from build123d import *

# Parameters (mm, degrees)
SKETCH1_W               = 355.6
SKETCH1_H               = 50.8
BOSS_EXTRUDE1_DEPTH     = 3.175
SKETCH2_W               = 38.1
SKETCH2_H               = 3.175
BOSS_EXTRUDE2_DEPTH     = 3.175
MIRROR2_COPY_1_SKETCH_W = 38.1
MIRROR2_COPY_1_SKETCH_H = 3.175
MIRROR2_COPY_1_DEPTH    = 3.175
SKETCH3_W               = 3.302
SKETCH3_H               = 26.67
CUT_EXTRUDE1_DEPTH      = 3.175
SKETCH4_R               = 1.4732
SKETCH4_R_2             = 12
SKETCH4_W               = 12.192
SKETCH4_H               = 12.192
CUT_EXTRUDE2_DEPTH      = 1
CUT_EXTRUDE2_DEPTH_BACK = 4.175


with BuildPart() as part:
    # Sketch1 → Boss-Extrude1 (new body)
    with BuildSketch(Plane.XY):
        with Locations((177.8, 25.4)):
            Rectangle(SKETCH1_W, SKETCH1_H)
    extrude(amount=BOSS_EXTRUDE1_DEPTH)

    # Sketch2 → Boss-Extrude2 (add)
    with BuildSketch(Plane(origin=(0, 50.8, 0), x_dir=(1, 0, 0), z_dir=(0, 1, 0))):
        with Locations((50.8, -1.5875)):
            Rectangle(SKETCH2_W, SKETCH2_H)
        with Locations((127, -1.5875)):
            Rectangle(SKETCH2_W, SKETCH2_H)
    boss_extrude2 = extrude(amount=BOSS_EXTRUDE2_DEPTH)

    # Mirror1: Boss-Extrude2 across plane
    add(boss_extrude2.mirror(Plane.ZY.offset(-177.8)))

    # Mirror2: Boss-Extrude2 across plane
    add(boss_extrude2.mirror(Plane.ZX.offset(25.4)))

    # Mirror2 copy 1 sketch → Mirror2 copy 1 (add)
    with BuildSketch(Plane(origin=(355.6, 0, 0), x_dir=(-1, 0, 0), z_dir=(0, -1, 0))):
        with Locations((50.8, -1.5875)):
            Rectangle(MIRROR2_COPY_1_SKETCH_W, MIRROR2_COPY_1_SKETCH_H)
        with Locations((127, -1.5875)):
            Rectangle(MIRROR2_COPY_1_SKETCH_W, MIRROR2_COPY_1_SKETCH_H)
    extrude(amount=MIRROR2_COPY_1_DEPTH)

    # Sketch3 → Cut-Extrude1 (cut)
    with BuildSketch(Plane(origin=(0, 0, 0), x_dir=(-1, 0, 0), z_dir=(0, 0, -1))):
        with Locations((-8.001, 13.335)):
            Rectangle(SKETCH3_W, SKETCH3_H)
    cut_extrude1 = extrude(amount=-CUT_EXTRUDE1_DEPTH, mode=Mode.SUBTRACT)

    # Mirror3: Cut-Extrude1 across plane
    add(cut_extrude1.mirror(Plane.ZY.offset(-177.8)), mode=Mode.SUBTRACT)

    # Sketch4 → Cut-Extrude2 (cut, two sides)
    with BuildSketch(Plane(origin=(0, 0, 0), x_dir=(-1, 0, 0), z_dir=(0, 0, -1))) as cut_extrude2_sk:
        with Locations((-220.9, 25.4)):
            Circle(SKETCH4_R)
        with Locations((-246.9, 25.4)):
            Circle(SKETCH4_R)
        with Locations((-292.1, 25.4)):
            Circle(SKETCH4_R_2)
        with Locations((-233.9, 25.4)):
            Rectangle(SKETCH4_W, SKETCH4_H)
    extrude(amount=CUT_EXTRUDE2_DEPTH, mode=Mode.SUBTRACT)
    extrude(cut_extrude2_sk.sketch, amount=-CUT_EXTRUDE2_DEPTH_BACK, mode=Mode.SUBTRACT)


solid = part.part
Geometry check sheet. Reference: the model listing, model coordinates, mm. Round coordinates to 2 decimals unless told otherwise and drop trailing zeros. Loops run counter-clockwise (first coordinate to the right, second up) from the corner with the lowest first, then second, coordinate; pieces in that order, holes last.
Item 1: Mould release check, pull along X, two halves, no side actions. Record for faces 1 (the flat face through (175, 26, 3.175)), 2 (the cylindrical face through (280.654, 29.004, 1.565)): pulls with the +X half, pulls with the -X half, needs draft (parallel to the pull), parting line crosses it, or undercut.
Item 2: Gauge pin test, flat ends, axial feed: pin 1 (1.6 mm diameter, centred on x = 351, z = 2.5, fed in from -Y); pin 2 (1.6 mm diameter, centred on x = 183.5, z = 2, fed in from +Y); pin 3 (1.6 mm diameter, centred on y = 52.5, z = 1.5, fed in from -X). Record the tip position at first contact, or that the pin passes through.
Item 3: Cross-section at A-A on x = 292.1. Record the boundary of the cut face in (y, z) (3 decimals), then the cut area to 3 significant figures.
Item 4: Cross-section at B-B on z = 0.7. Count the separate pieces of the cut face and the enclosed holes in it, then the cut area to 3 significant figures.
Item 5: Thickness scan on line 1 (X direction, y = 2.5, z = 2.9); line 2 (Y direction, x = 231.5, z = 1.2) (3 decimals); line 3 (Y direction, x = 220.9, z = 1.75) (3 decimals). Record the ranges inside material, lowest first.
Item 6: Cross-section at C-C on x = 28. Record the boundary of the cut face in (y, z) (3 decimals), then the cut area to 3 significant figures.
Answer sheet:
1. face 1: needs draft
1. face 2: undercut
2. pin 1: stops at y = 0
2. pin 2: stops at y = 50.8
2. pin 3: stops at x = 31.75
3. outline: (-3.175, 0) - (13.4, 0) - (13.4, 3.175) - (-3.175, 3.175) - close; (37.4, 0) - (53.975, 0) - (53.975, 3.175) - (37.4, 3.175) - close
3. area: 105 mm2
4. separate pieces: 1
4. enclosed holes: 4
4. area: 18,200 mm2
5. line 1: x = 0 to 6.35, 9.65 to 345.95, 349.25 to 355.6
5. line 2: y = -3.175 to 19.304, 31.496 to 53.975
5. line 3: y = -3.175 to 23.927, 26.873 to 53.975
6. outline: (0, 0) - (50.8, 0) - (50.8, 3.175) - (0, 3.175) - close
6. area: 161 mm2
